Drawing for the job (mm, zero at the part's lowest x, y, z). A direction names the side the tool comes from. Coordinates: 2 decimals unless noted, no trailing zeros. Order: outer loops, then holes, each group sorted by start corner. A loop starts at its lowest first (then second) coordinate and runs counter-clockwise, first axis right, second up. Notation, with made-up numbers: M 54.25,18.5 L 98.25,18.5 A22 cw 98.25,34.5 Z; hole C 81.5,3.5 d4. An arc over 180 degrees is marked long. Write item = value, one per line. Start each with the question number.
Q1. Pin check, flat tip, straight feed: P1, Ø4, axis at y = 120.5, z = 37, coming from the -X side. Stop position of the tip, or through.
Q2. Band-saw the part on B-B on z = 17. Write the cut outline in (x, y).
Q3. Pull direction Y, two halves, no side cores. Call the marked faces 3, 4 and 5: released by +Y, released by -Y, zero draft, split by the parting line, or undercut.
Q4. Band-saw the part on A-A on y = 125. Write the cut outline in (x, z).
Q5. 3-axis set-ups, long thin cutter, end or side, ignore diameter. For the marked faces 1 and 2: which of +Z, -Z, +X, -X, +Y, -Y reach the whole face in a straight line?
Q6. Drill centre line: probe 1 along X at (y, z) = (147, 32). Where is it in solid material? Low to high.
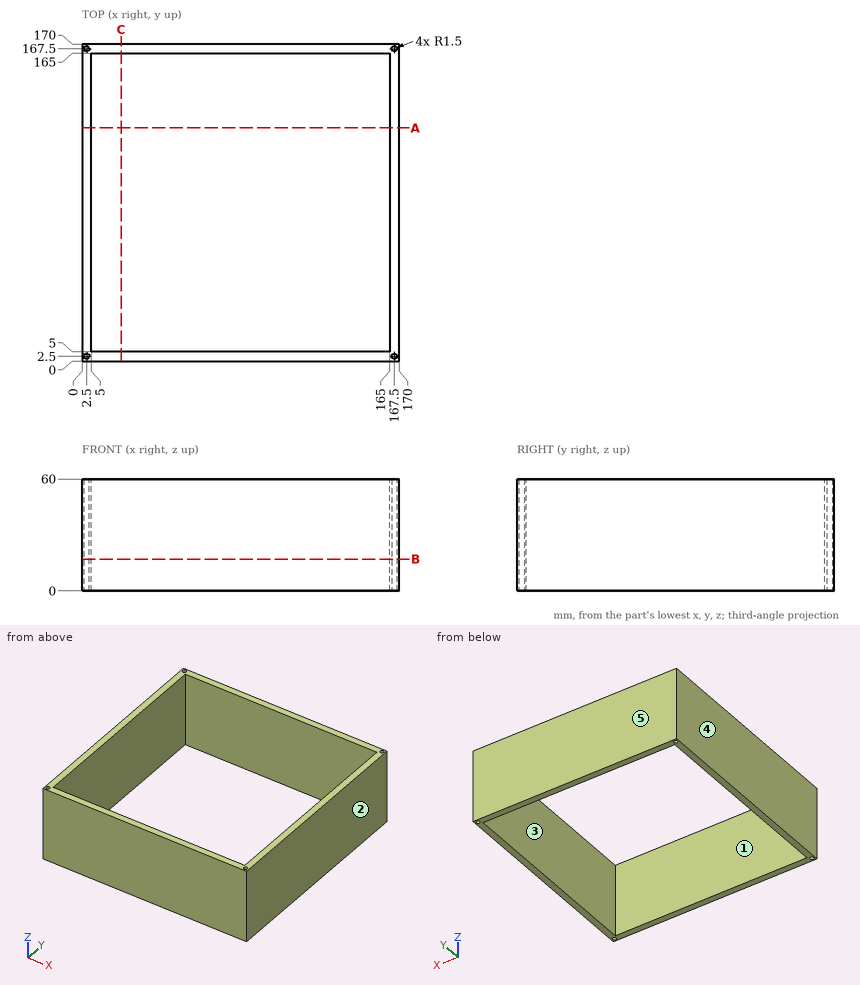
Recorded:
q1.P1 = 0
q2.outline = M 0,0 L 170,0 L 170,170 L 0,170 Z; hole M 1.44,1.44 A1.5 ccw 4,2.5 A1.5 ccw 3.56,3.56 A1.5 ccw Z; hole M 1.44,168.56 A1.5 ccw 3.56,166.44 A1.5 ccw 4,167.5 A1.5 ccw Z; hole M 5,5 L 165,5 L 165,165 L 5,165 Z; hole M 168.56,1.44 A1.5 ccw 169,2.5 A1.5 ccw long Z; hole M 168.56,168.56 A1.5 ccw long 169,167.5 A1.5 ccw Z
q3.face_3 = undercut
q3.face_4 = zero draft
q3.face_5 = released by +Y
q4.outline = M 0,0 L 5,0 L 5,60 L 0,60 Z; M 165,0 L 170,0 L 170,60 L 165,60 Z
q5.face_1 = +Z, -Z
q5.face_2 = +Z, -Z, +X, +Y, -Y
q6.probe_1 = 0 to 5, 165 to 170
